from build123d import *

# Parameters (mm, degrees)
F0_W     = 30
F0_H     = 150
F0_R     = 8.5
F1_DEPTH = 8
F2_R     = 5
F3_DEPTH = 15
F4_R     = 5
F5_DEPTH = 15
F6_R     = 1.15
F7_DEPTH = 25


with BuildPart() as f1:
    # F0 (on Top) → F1 (new body)
    with BuildSketch(Plane.XY):
        with Locations((18.116215, -75)):
            Rectangle(F0_W, F0_H)
        with Locations((18.116215, -20.311708)):
            Circle(F0_R, mode=Mode.SUBTRACT)
    extrude(amount=F1_DEPTH)

    # F2 (on face) → F3 (join)
    with BuildSketch(Plane.XY.offset(8)):
        with Locations((18.116215, -85.969344)):
            Circle(F2_R)
    extrude(amount=F3_DEPTH)

    # F4 (on face) → F5 (join)
    with BuildSketch(Plane(origin=(0, 0, 0), x_dir=(1, 0, 0), z_dir=(0, 0, -1))):
        with Locations((18.116215, 87.31737)):
            Circle(F4_R)
    extrude(amount=F5_DEPTH)

    # F6 (on face) → F7 (cut)
    with BuildSketch(Plane(origin=(0, 0, 0), x_dir=(1, 0, 0), z_dir=(0, 0, -1))):
        with Locations((18.116215, 142.368332)):
            Circle(F6_R)
    extrude(amount=-F7_DEPTH, mode=Mode.SUBTRACT)


solid = f1.part
Could you check a few things on this model? Use its own coordinates, in mm. A direction names the side the tool comes from. Coordinates: 2 decimals unless noted, no trailing zeros. Loops run counter-clockwise (first coordinate to the right, second up) from the corner with the lowest first, then second, coordinate; pieces in that order, holes last.
1. Imagine slicing it at A-A (x = 21). Please give me the cut outline in (y, z).
2. Imagine slicing it at D-D (x = 28.75). Please give me the cut outline in (y, z).
3. Imagine slicing it at B-B (y = -23). Please give me the cut outline in (x, z).
4. For P1, Ø1.5, axis at x = 24.5, y = -27.5, coming from the +Z side; P2, Ø1, axis at x = 11.5, y = -71, coming from the -Z side; P3, Ø4, axis at x = 20.5, z = 14, coming from the -Y side, each with a flat end and sliding along its axis, tell me the tip position at first contact or that it passes through.
5. I need wall thicknesses on L1, parallel to Z at x = 30, y = -53; L2, parallel to X at y = -18, z = 5; L3, parallel to X at y = -87.5, z = -4.5. Which ranges of each line are inside material? Lowest first, please.
6. We'd pull the mould along X, two halves only. Please class faces 1 (the face through (16.27, -28.61, 3.94)), 2 (the face through (3.116, -76, 4)), 3 (the face through (18, -74, 0)): released by +X, released by -X, zero draft, split by the parting line, or undercut.
7. Imagine slicing it at C-C (z = 6.5). Please give me the cut outline in (x, y).
8. For faces 4 (the face through (17.032, -82.436, -7.395)), 5 (the face through (17.03, -90.85, 15.4)), 6 (the face through (18, -150, 4)), which set-ups out of +Z, -Z, +X, -X, +Y, -Y let a thin tool reach every point of the face, with its end or its side?
Computed values:
1. outline: (-150, 0) - (-91.4, 0) - (-91.4, -15) - (-83.23, -15) - (-83.23, 0) - (-28.31, 0) - (-28.31, 8) - (-81.88, 8) - (-81.88, 23) - (-90.05, 23) - (-90.05, 8) - (-150, 8) - close; (-12.32, 0) - (0, 0) - (0, 8) - (-12.32, 8) - close
2. outline: (-150, 0) - (0, 0) - (0, 8) - (-150, 8) - close
3. outline: (3.12, 0) - (10.05, 0) - (10.05, 8) - (3.12, 8) - close; (26.18, 0) - (33.12, 0) - (33.12, 8) - (26.18, 8) - close
4. P1: stops at z = 8
4. P2: stops at z = 0
4. P3: stops at y = -90.95
5. L1: z = 0 to 8
5. L2: x = 3.12 to 9.94, 26.3 to 33.12
5. L3: x = 13.12 to 23.11
6. face 1: undercut
6. face 2: released by -X
6. face 3: zero draft
7. outline: (3.12, -150) - (33.12, -150) - (33.12, 0) - (3.12, 0) - close; hole circle Ø17 at (18.12, -20.31); hole circle Ø2.3 at (18.12, -142.37)
8. face 4: -Z
8. face 5: +Z
8. face 6: +Z, -Z, +X, -X, -Y
